```python
from build123d import *

# Parameters (mm, degrees)
F2_R     = 5
F7_D     = 5
F7_DEPTH = 6
F7_TIP   = 1.5021515476
F8_R     = 5


with BuildPart() as f3:
    # F3: sweep along a path in F0
    with BuildLine(Plane.XZ) as f3_path:
        Line((60, 0), (2.307932585, 0))
        ThreePointArc((2.307932585, 0), (0.212461852, 0.4602860875), (-1.497202471, 1.7563990372))
        Line((-1.497202471, 1.7563990372), (-38.4974752497, 45.1621806509))
    # F2 (on offset) → F3 (sweep)
    with BuildSketch(Plane.YZ.offset(60)):
        Circle(F2_R)
    sweep(path=f3_path.line)

    # F7
    with Locations(Plane.XY.offset(5)):
        with Locations((35.039074719, 0)):
            Hole(F7_D / 2, depth=F7_DEPTH)
            with Locations((0, 0, -(F7_DEPTH + F7_TIP / 2))):  # 118° drill point
                Cone(0, F7_D / 2, F7_TIP, mode=Mode.SUBTRACT)

    # F8
    f8_edges = [f3.edges().sort_by_distance(p)[0] for p in [
        (-38.497475, -5, 45.162181),
    ]]
    fillet(f8_edges, radius=F8_R)


solid = f3.part
```
Build history of the part. All positions in model axes, mm. A direction names the side the tool comes from. Give positions to 0.01 mm unless a question says otherwise; leave off trailing zeros. Order: outer loops, then holes, each group sorted by start corner. A loop starts at its lowest first (then second) coordinate and runs counter-clockwise, first axis right, second up. Notation, with made-up numbers: M 13,-32 L 48,-32 A17 ccw 48,-9 Z; hole C 31.25,55.5 d7. An arc over 180 degrees is marked long. Write item = value, one per line. Start each with the question number.
(1) Which spindle directions (+Z, -Z, +X, -X, +Y, -Y) get a long thin tool onto all of the face, cutting with end or side? Do faces 4 (the conical face through (35.44, -0.17, -2.24)), 5 (the cylindrical face through (31, 3, -4)). Say none if no direction does.
(2) Probe L1, parallel to Z at x = 25, y = 0; L2, parallel to X at y = 0, z = 2; L3, parallel to X at y = 0, z = 3.5. List the from-to ranges inside material, lowest first. Write a range as [from, to].
(3) Slice it at A-A on x = 13. Write the cut outline in (y, z), plus the area to 3 significant figures.
(4) Pin check, flat tips, straight feed: pin 1 Ø5 at (x, z) = (1.5, 4) entering from -Y; pin 2 Ø6 at (y, z) = (-1, 3.5) entering from -X; pin 3 Ø2 at (y, z) = (-3, 40) entering from -X. Stop position of each tip, or through.
(5) Two-plate mould, pull along X, no slides. Class faces 1 (the cylindrical face through (37.537, 0.11, 1.958)), 2 (the cylindrical face through (-14.9, -1.1, 25)), 3 (the flat face through (60, 0, 0)): released by +X, released by -X, zero draft, split by the parting line, or undercut.
Responses:
q1.face_4 = +Z
q1.face_5 = +X
q2.L1 = [-5, 5]
q2.L2 = [-8.27, 32.54], [37.54, 60]
q2.L3 = [-9.55, 32.54], [37.54, 60]
q3.outline = C 0,0 d10
q3.area = 78.5 mm2
q4.pin_1 = -4.85
q4.pin_2 = -12.04
q4.pin_3 = -39.7
q5.face_1 = undercut
q5.face_2 = split by the parting line
q5.face_3 = released by +X
